Input: part model. Units: mm. Frame: model coordinates. Face numbers are marked on the shaded views. A direction names the side the tool comes from. Round coordinates to 2 decimals unless told otherwise and drop trailing zeros. Write each loop counter-clockwise with the first axis right and the second up, starting at its lowest first coordinate (ties: lowest second). Pieces come first, ordered by that corner, then holes. Notation, with made-up numbers: (-37.5, 76) -> (-10.5, 76) arc R17 cw to (-10.5, 102) -> close; hole circle Ø6 at (-1, 76). An arc over 180 degrees is marked (long way). Use CSV: the item, a comma, the result in double quotes.
```python
from build123d import *
from build123d.topology import SkipClean

# Parameters (mm, degrees)
SKETCH1_R           = 32
SKETCH1_R_2         = 22.5
SKETCH3_R           = 60
SKETCH3_R_2         = 22.5
BOSS_EXTRUDE1_DEPTH = 20
BOSS_EXTRUDE2_START = 20
SKETCH4_R           = 60
SKETCH4_R_2         = 22.5
BOSS_EXTRUDE2_DEPTH = 20
HOLE1_D             = 15
HOLE1_DEPTH         = 20
CIRPATTERN1_COUNT   = 4
HOLE2_D             = 15
HOLE2_DEPTH         = 20
CIRPATTERN2_COUNT   = 4
SKETCH12_R          = 12
BOSS_EXTRUDE3_DEPTH = 20
BOSS_EXTRUDE4_DEPTH = 12
SKETCH21_W          = 64
SKETCH21_H          = 81.283369249
BOSS_EXTRUDE5_DEPTH = 10


with BuildPart() as part:
    # Sweep1: sweep along a path in Sketch2
    with BuildLine(Plane(origin=(0, 0, 0), x_dir=(0, 0, -1), z_dir=(1, 0, 0))) as sweep1_path:
        Line((0, 0), (200, 0))
        ThreePointArc((200, 0), (256.568542495, 23.431457505), (280, 80))
        Line((280, 80), (280, 205))
    # Sketch1 → Sweep1 (sweep)
    with BuildSketch(Plane.XY):
        Circle(SKETCH1_R)
        Circle(SKETCH1_R_2, mode=Mode.SUBTRACT)
    sweep(path=sweep1_path.line)

    # Sketch3 → Boss-Extrude1 (add)
    with SkipClean():  # the faces are left unmerged after this step: merging them gives an invalid solid
        with BuildSketch(Plane.XY):
            Circle(SKETCH3_R)
            with Locations(Location((0, 0, 0), (0, 0, 270))):
                Circle(SKETCH3_R_2, mode=Mode.SUBTRACT)
        extrude(amount=BOSS_EXTRUDE1_DEPTH)

    # Sketch4 → Boss-Extrude2 (add)
    with SkipClean():  # the faces are left unmerged after this step: merging them gives an invalid solid
        with BuildSketch(Plane(origin=(0, 205, 0), x_dir=(1, 0, 0), z_dir=(0, 1, 0)).offset(BOSS_EXTRUDE2_START)):
            with Locations(Location((0, 280, 0), (0, 0, 270))):
                Circle(SKETCH4_R)
            with Locations(Location((0, 280, 0), (0, 0, 270))):
                Circle(SKETCH4_R_2, mode=Mode.SUBTRACT)
        extrude(amount=-BOSS_EXTRUDE2_DEPTH)

    # Hole1
    with Locations(Plane.XY.offset(20)):
        with Locations((45, 0)):
            hole1 = Hole(HOLE1_D / 2, depth=HOLE1_DEPTH)

    # CirPattern1: Hole1 ×4 about axis
    with SkipClean():  # the faces are left unmerged after this step: merging them gives an invalid solid
        cirpattern1_axis = Axis((0, 0, 0), (0, 0, 1))
        for i in range(1, CIRPATTERN1_COUNT):
            add(hole1.rotate(cirpattern1_axis, i * 360 / CIRPATTERN1_COUNT), mode=Mode.SUBTRACT)

    # Hole2
    with Locations(Plane(origin=(0, 225, 0), x_dir=(1, 0, 0), z_dir=(0, 1, 0))):
        with Locations((0, 235)):
            hole2 = Hole(HOLE2_D / 2, depth=HOLE2_DEPTH)

    # CirPattern2: Hole2 ×4 about axis
    with SkipClean():  # the faces are left unmerged after this step: merging them gives an invalid solid
        cirpattern2_axis = Axis((0, 0, -280), (0, 1, 0))
        for i in range(1, CIRPATTERN2_COUNT):
            add(hole2.rotate(cirpattern2_axis, i * 360 / CIRPATTERN2_COUNT), mode=Mode.SUBTRACT)



with BuildPart() as body_2:
    # Sketch12 → Boss-Extrude3 (new body)
    with BuildSketch(Plane(origin=(0, -120, 0), x_dir=(1, 0, 0), z_dir=(0, 1, 0))):
        with BuildLine():
            Line((10.714285714, 97.705881545), (99.857142857, 75.852940773))
            ThreePointArc((99.857142857, 75.852940773), (117, 54), (99.857142857, 32.147059227))
            Line((99.857142857, 32.147059227), (10.714285714, 10.294118455))
            ThreePointArc((10.714285714, 10.294118455), (0, 9), (-10.714285714, 10.294118455))
            Line((-10.714285714, 10.294118455), (-99.857142857, 32.147059227))
            ThreePointArc((-99.857142857, 32.147059227), (-117, 54), (-99.857142857, 75.852940773))
            Line((-99.857142857, 75.852940773), (-10.714285714, 97.705881545))
            ThreePointArc((-10.714285714, 97.705881545), (0, 99), (10.714285714, 97.705881545))
        make_face()
        with Locations(Location((-94.5, 54, 0), (0, 0, 270))):
            Circle(SKETCH12_R, mode=Mode.SUBTRACT)
        with Locations(Location((94.5, 54, 0), (0, 0, 270))):
            Circle(SKETCH12_R, mode=Mode.SUBTRACT)
    extrude(amount=BOSS_EXTRUDE3_DEPTH)


with BuildPart() as part_1:
    with SkipClean():  # the faces are left unmerged after this step: merging them gives an invalid solid
        add(part.part)

        add(body_2.part)  # Boss-Extrude4 merges body 2
        # Sketch19 → Boss-Extrude4 (add, symmetric)
        with BuildSketch(Plane.XY.offset(-54)):
            with BuildLine():
                Line((21.348386826, 7.106080491), (57, -100))
                Line((57, -100), (-57, -100))
                Line((-57, -100), (-21.348386826, 7.106080491))
                ThreePointArc((-21.348386826, 7.106080491), (0, -22.5), (21.348386826, 7.106080491))
            make_face()
        extrude(amount=BOSS_EXTRUDE4_DEPTH, both=True)

    # Sketch21 → Boss-Extrude5 (add, symmetric)
    with SkipClean():  # the faces are left unmerged after this step: merging them gives an invalid solid
        with BuildSketch(Plane(origin=(0, 0, 0), x_dir=(0, 0, -1), z_dir=(1, 0, 0))):
            with Locations((54, -65.842294917)):
                Rectangle(SKETCH21_W, SKETCH21_H)
        extrude(amount=BOSS_EXTRUDE5_DEPTH, both=True)


solid = part_1.part
```
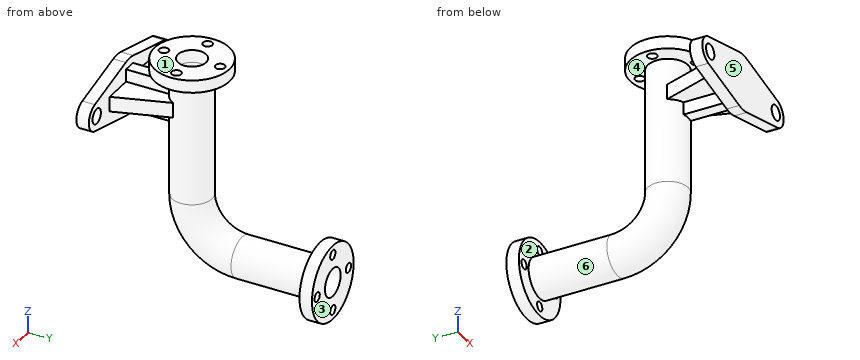
Item 1: First-contact query: pin 1 Ø2 at (y, z) = (173.5, -290.5) entering from +X; pin 2 Ø8 at (y, z) = (79.5, -243.5) entering from -X; pin 3 Ø16 at (y, z) = (-55.5, -35.5) entering from -X; pin 4 Ø16 at (y, z) = (-68.5, -79) entering from -X. Flat tips, straight axial feed; report the tip coordinate or a pass-through.
Worked answers:
pin 1,"stops at x = 30.56"
pin 2,"passes through"
pin 3,"stops at x = -43.74"
pin 4,"stops at x = -10"
Item 2: Set-up query: the marked faces 1 and 2. Return all of +Z, -Z, +X, -X, +Y, -Y with unobstructed straight access to the full face (end or side cutting, diameter ignored); none if empty.
Worked answers:
face 1,"+Z, +X, -X, +Y, -Y"
face 2,"none"
Item 3: Section query C-C on x = 45. Return the cut outline in (y, z).
Worked answers:
outline,"(-120, -89.3) -> (-100, -89.3) -> (-100, -66) -> (-63.95, -66) -> (-63.95, -42) -> (-100, -42) -> (-100, -18.7) -> (-120, -18.7) -> close; (-39.69, 0) -> (-7.5, 0) -> (-7.5, 20) -> (-39.69, 20) -> close; (7.5, 0) -> (39.69, 0) -> (39.69, 20) -> (7.5, 20) -> close; (205, -319.69) -> (225, -319.69) -> (225, -287.5) -> (205, -287.5) -> close; (205, -272.5) -> (225, -272.5) -> (225, -240.31) -> (205, -240.31) -> close"
Item 4: Section query D-D on y = -45. Return the cut outline in (x, z).
Worked answers:
outline,"(-39.69, 0) -> (-7.5, 0) -> (-7.5, 20) -> (-39.69, 20) -> close; (-38.69, -66) -> (-10, -66) -> (-10, -86) -> (10, -86) -> (10, -66) -> (38.69, -66) -> (38.69, -42) -> (10, -42) -> (10, -22) -> (-10, -22) -> (-10, -42) -> (-38.69, -42) -> close; (7.5, 0) -> (39.69, 0) -> (39.69, 20) -> (7.5, 20) -> close"
Item 5: Section query A-A on z = -54. Return the cut outline in (x, y).
Worked answers:
outline,"(-117, -120) -> (-106.5, -120) -> (-106.5, -100) -> (-117, -100) -> close; (-82.5, -120) -> (82.5, -120) -> (82.5, -100) -> (57, -100) -> (28.53, -14.48) arc R32 ccw (long way) to (-28.53, -14.48) -> (-57, -100) -> (-82.5, -100) -> close; (106.5, -120) -> (117, -120) -> (117, -100) -> (106.5, -100) -> close; hole circle Ø45 at (0, 0)"
Item 6: Section query B-B on x = -94.5. Return the cut outline in (y, z).
Worked answers:
outline,"(-120, -77.17) -> (-100, -77.17) -> (-100, -66) -> (-120, -66) -> close; (-120, -42) -> (-100, -42) -> (-100, -30.83) -> (-120, -30.83) -> close"
Item 7: Pull-direction query (Y, two-part tool) for the marked faces 3, 4, 5 and 6; classes: +Y half, -Y half, draft (parallel to the pull), parting line (faces both ways), or undercut.
Worked answers:
face 3,"+Y half"
face 4,"draft"
face 5,"-Y half"
face 6,"undercut"
Item 8: Line query: line 1 (X direction, y = -112.5, z = -54); line 2 (X direction, y = 0, z = -84.5). Output: solid intervals per line, ascending.
Worked answers:
line 1,"x = -117 to -106.5, -82.5 to 82.5, 106.5 to 117"
line 2,"x = -32 to -22.5, 22.5 to 32"
